Part print with two shaded views. Sizes in mm from the minimum x, y, z corner. Round coordinates to 2 decimals unless told otherwise and drop trailing zeros. Loops run counter-clockwise (first coordinate to the right, second up) from the corner with the lowest first, then second, coordinate; pieces in that order, holes last. Notation, with made-up numbers: (65.5, 61.25) -> (79.5, 61.25) arc R36 cw to (79.5, 96.25) -> close; hole circle Ø1 at (27.5, 88). An arc over 180 degrees is marked (long way). Use a Markdown table: item, result. Add a question column.
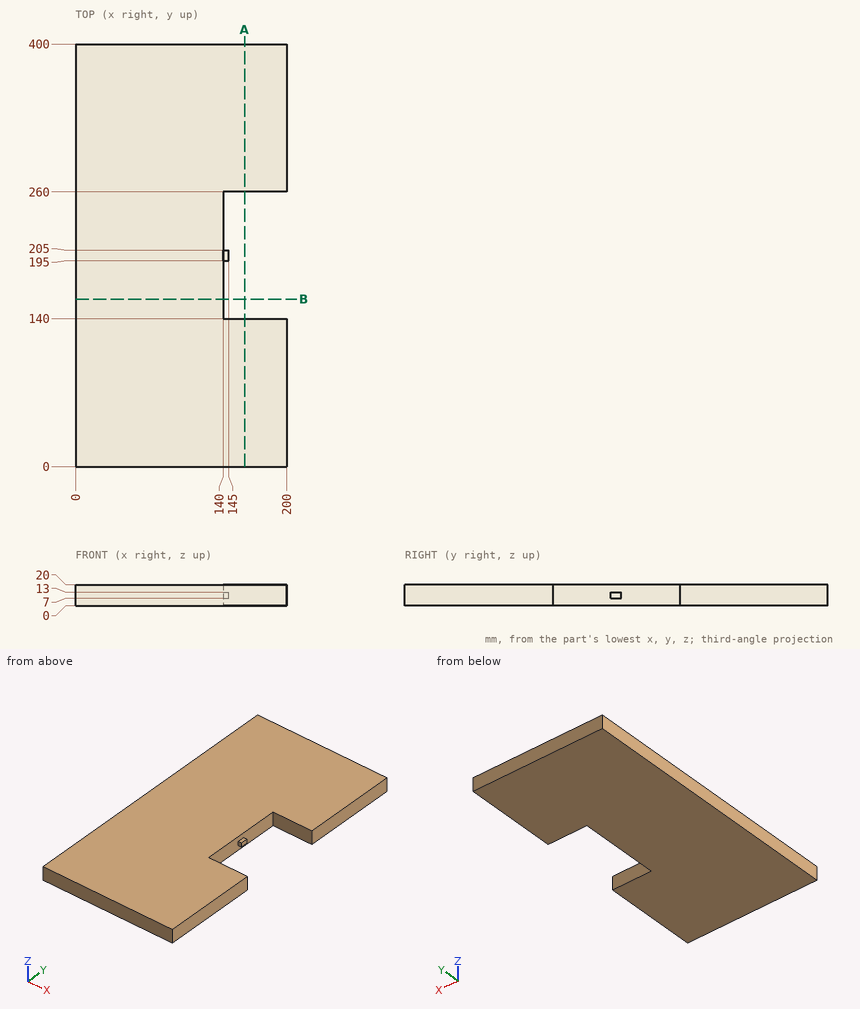
1) Wall check: probe 1 along Y at (x, z) = (143, 3.25); probe 2 along X at (y, z) = (215, 10.75). Give the ranges that are in metal, low to high. Write a range as from..to.
2) Cut at A-A on x = 160. Write the cut outline in (y, z).
3) Cut at B-B on y = 158.5. Write the cut outline in (x, z).
4) Pin check, flat tips, straight feed: pin 1 Ø5 at (y, z) = (201, 10) entering from +X; pin 2 Ø5.5 at (x, y) = (143, 200) entering from -Z; pin 3 Ø10 at (y, z) = (232.5, 4) entering from +X. Stop position of each tip, or through.
Established:
| question | item | result |
|---|---|---|
| 1 | probe 1 | y = 0..140, 260..400 |
| 1 | probe 2 | x = 0..140 |
| 2 | outline | (0, 0) -> (140, 0) -> (140, 20) -> (0, 20) -> close; (260, 0) -> (400, 0) -> (400, 20) -> (260, 20) -> close |
| 3 | outline | (0, 0) -> (140, 0) -> (140, 20) -> (0, 20) -> close |
| 4 | pin 1 | stops at x = 145 |
| 4 | pin 2 | stops at z = 7 |
| 4 | pin 3 | stops at x = 140 |
